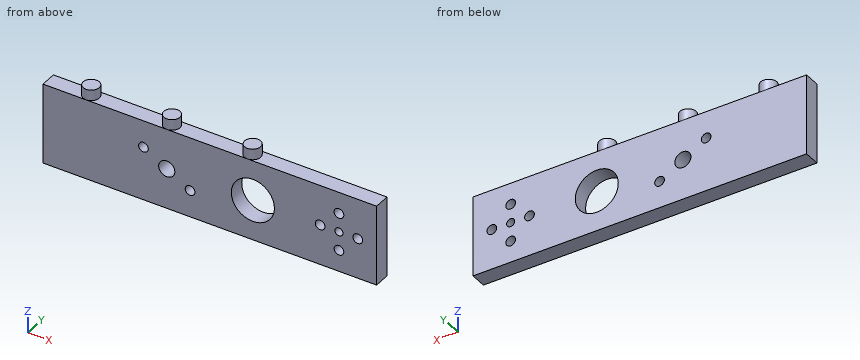
from build123d import *

# Parameters (mm, degrees)
SKETCH_1_W      = 62
SKETCH_1_H      = 15
SKETCH_1_R      = 1.5
SKETCH_1_R_2    = 0.9
SKETCH_1_R_3    = 4
SKETCH_1_R_4    = 0.75
EXTRUDE_1_DEPTH = 3
SKETCH_2_R      = 1.5
EXTRUDE_2_DEPTH = 2


with BuildPart() as part:
    # 草图1 → 凸台-拉伸1 (new body)
    with BuildSketch(Plane(origin=(0, 0, 0), x_dir=(1, 0, 0), z_dir=(0, 1, 0))):
        Rectangle(SKETCH_1_W, SKETCH_1_H)
        with Locations(Location((-8, 0, 0), (0, 0, 270))):
            Circle(SKETCH_1_R, mode=Mode.SUBTRACT)
        with Locations(Location((-3.669872981, 2.5, 0), (0, 0, 270))):
            Circle(SKETCH_1_R_2, mode=Mode.SUBTRACT)
        with Locations(Location((-12.330127019, -2.5, 0), (0, 0, 270))):
            Circle(SKETCH_1_R_2, mode=Mode.SUBTRACT)
        with Locations(Location((8, 0, 0), (0, 0, 270))):
            Circle(SKETCH_1_R_3, mode=Mode.SUBTRACT)
        with Locations(Location((24, 0, 0), (0, 0, 270))):
            Circle(SKETCH_1_R_4, mode=Mode.SUBTRACT)
        with Locations(Location((27.5, 0, 0), (0, 0, 270))):
            Circle(SKETCH_1_R_2, mode=Mode.SUBTRACT)
        with Locations(Location((24, -3.5, 0), (0, 0, 270))):
            Circle(SKETCH_1_R_2, mode=Mode.SUBTRACT)
        with Locations(Location((20.5, 0, 0), (0, 0, 270))):
            Circle(SKETCH_1_R_2, mode=Mode.SUBTRACT)
        with Locations(Location((24, 3.5, 0), (0, 0, 270))):
            Circle(SKETCH_1_R_2, mode=Mode.SUBTRACT)
    extrude(amount=EXTRUDE_1_DEPTH)

    # 草图2 → 凸台-拉伸2 (add)
    with BuildSketch(Plane.XY.offset(7.5)):
        with Locations(Location((-23, 1.5, 0), (0, 0, 270))):
            Circle(SKETCH_2_R)
        with Locations(Location((-8, 1.5, 0), (0, 0, 270))):
            Circle(SKETCH_2_R)
        with Locations(Location((7, 1.5, 0), (0, 0, 270))):
            Circle(SKETCH_2_R)
    extrude(amount=EXTRUDE_2_DEPTH)


solid = part.part
Build history of the part. All positions in model axes, mm. Round coordinates to 2 decimals unless told otherwise and drop trailing zeros. Loops run counter-clockwise (first coordinate to the right, second up) from the corner with the lowest first, then second, coordinate; pieces in that order, holes last. Notation, with made-up numbers: (74, 42) -> (95, 42) arc R26 ccw to (95, 79) -> close; hole circle Ø4 at (-30.75, 5.5). An arc over 180 degrees is marked (long way). Use CSV: the item, a comma, the result in double quotes. Start each with the question number.
Q1. Saw through at D-D on y = 1.5. Count the separate pieces of the cut face and the enclosed holes in it, and give its area (3 significant figures).
Q2. Drill centre lines: L1, parallel to X at y = 2.3, z = 0; L2, parallel to X at y = 2.25, z = 3.5; L3, parallel to X at y = 0.8, z = -2.5. Where is each one in solid material? Low to high.
Q3. Saw through at C-C on z = 8.5. Give the cut face in (x, y).
Q4. Flat gauge pins, fed straight in: pin 1 Ø1.4 at (x, z) = (24, 3.5) entering from -Y; pin 2 Ø1.5 at (x, z) = (-2.5, -3) entering from -Y; pin 3 Ø0.9 at (x, y) = (-27.5, 2) entering from +Z. Where does each tip first touch, or does it go through?
Q5. Saw through at B-B on x = 27.5. Give the cut face in (y, z), and give its area (3 significant figures).
Q6. Saw through at A-A on z = 0. Give the cut face in (x, y), and give its area (3 significant figures).
Solutions:
1,separate pieces,"1"
1,enclosed holes,"9"
1,area,"874 mm^2"
2,L1,"x = -31 to -9.5, -6.5 to 4, 12 to 19.6, 21.4 to 23.25, 24.75 to 26.6, 28.4 to 31"
2,L2,"x = -31 to 6.06, 9.94 to 23.1, 24.9 to 31"
2,L3,"x = -31 to -4.57, -2.77 to 4.88, 11.12 to 31"
3,outline,"circle Ø3 at (-23, 1.5); circle Ø3 at (-8, 1.5); circle Ø3 at (7, 1.5)"
4,pin 1,"passes through"
4,pin 2,"stops at y = 0"
4,pin 3,"stops at z = 7.5"
5,outline,"(0, -7.5) -> (3, -7.5) -> (3, -0.9) -> (0, -0.9) -> close; (0, 0.9) -> (3, 0.9) -> (3, 7.5) -> (0, 7.5) -> close"
5,area,"39.6 mm^2"
6,outline,"(-31, 0) -> (-9.5, 0) -> (-9.5, 3) -> (-31, 3) -> close; (-6.5, 0) -> (4, 0) -> (4, 3) -> (-6.5, 3) -> close; (12, 0) -> (19.6, 0) -> (19.6, 3) -> (12, 3) -> close; (21.4, 0) -> (23.25, 0) -> (23.25, 3) -> (21.4, 3) -> close; (24.75, 0) -> (26.6, 0) -> (26.6, 3) -> (24.75, 3) -> close; (28.4, 0) -> (31, 0) -> (31, 3) -> (28.4, 3) -> close"
6,area,"138 mm^2"
